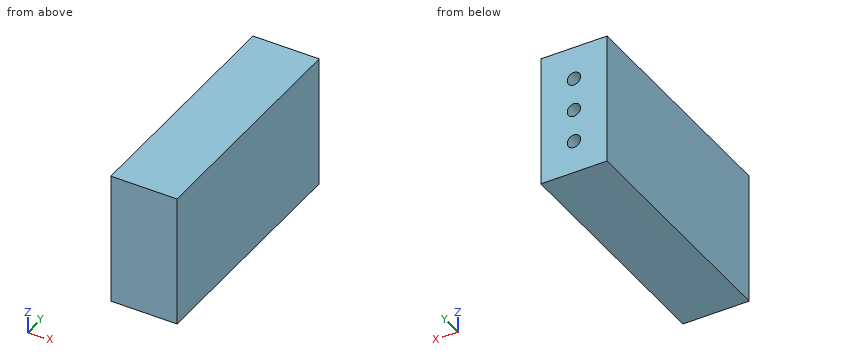
```python
from build123d import *

# Parameters (mm, degrees)
SKETCH1_W                   = 25.4
SKETCH1_H                   = 50.8
BOSS_EXTRUDE1_DEPTH         = 92.075
F_1_4_20_TAPPED_HOLE3_D     = 5.1054
F_1_4_20_TAPPED_HOLE3_DEPTH = 16.51
F_1_4_20_TAPPED_HOLE3_TIP   = 1.533816902


with BuildPart() as part:
    # Sketch1 → Boss-Extrude1 (new body)
    with BuildSketch(Plane(origin=(0, 0, 0), x_dir=(1, 0, 0), z_dir=(0, 1, 0))):
        Rectangle(SKETCH1_W, SKETCH1_H)
    extrude(amount=BOSS_EXTRUDE1_DEPTH)

    # 1/4-20 Tapped Hole3
    with Locations(Plane(origin=(0, 92.075, 0), x_dir=(1, 0, 0), z_dir=(0, 1, 0))):
        with Locations((0, 12.7), (0, 0), (0, -12.7)):
            Hole(F_1_4_20_TAPPED_HOLE3_D / 2, depth=F_1_4_20_TAPPED_HOLE3_DEPTH)
            with Locations((0, 0, -(F_1_4_20_TAPPED_HOLE3_DEPTH + F_1_4_20_TAPPED_HOLE3_TIP / 2))):  # 118° drill point
                Cone(0, F_1_4_20_TAPPED_HOLE3_D / 2, F_1_4_20_TAPPED_HOLE3_TIP, mode=Mode.SUBTRACT)


solid = part.part
```
Verification items for the finished model (mm, model axes). Give positions to 0.01 mm unless a question says otherwise; leave off trailing zeros. Loops run counter-clockwise (first coordinate to the right, second up) from the corner with the lowest first, then second, coordinate; pieces in that order, holes last.
1. Go/stop test with a flat-tipped pin: pin 1 Ø6.5 at (x, z) = (0, -12.7) entering from +Y (3 decimals). Record where the tip stops, or that it passes through.
2. Section check A-A, the plane y = 79.5. Enter the section's corners in (x, z).
3. Thickness scan on line 1 (Z direction, x = 0, y = 86.25); line 2 (X direction, y = 86, z = 12); line 3 (Y direction, x = -0.75, z = 0.5). Record the ranges inside material, lowest first.
Geometry says:
1. pin 1: stops at y = 92.075
2. outline: (-12.7, -25.4) - (12.7, -25.4) - (12.7, 25.4) - (-12.7, 25.4) - close; hole circle Ø5.11 at (0, -12.7); hole circle Ø5.11 at (0, 0); hole circle Ø5.11 at (0, 12.7)
3. line 1: z = -25.4 to -15.25, -10.15 to -2.55, 2.55 to 10.15, 15.25 to 25.4
3. line 2: x = -12.7 to -2.45, 2.45 to 12.7
3. line 3: y = 0 to 74.57
